Geometry check sheet. Reference: the model listing, model coordinates, mm. Face numbers are marked on the shaded views. Coordinates: 2 decimals unless noted, no trailing zeros. Loops run counter-clockwise (first coordinate to the right, second up) from the corner with the lowest first, then second, coordinate; pieces in that order, holes last.
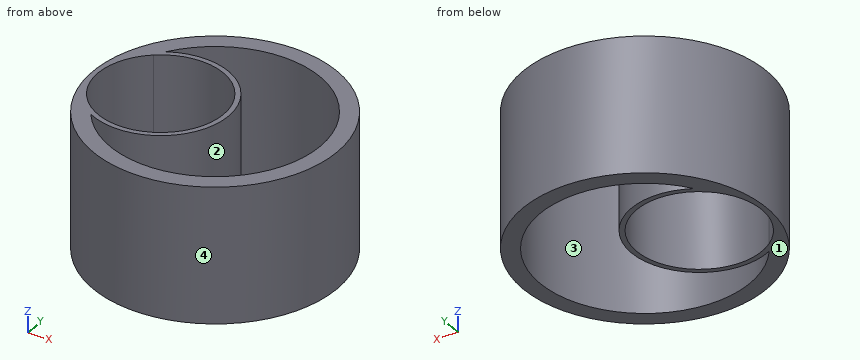
Autodesk Inventor part; units mm, degrees
ref_plane "YZ Plane" through (0, 0, 0) normal (1, 0, 0) x (0, 1, 0)
ref_plane "XZ Plane" through (0, 0, 0) normal (0, 1, 0) x (-1, 0, 0)
ref_plane "XY Plane" through (0, 0, 0) normal (0, 0, 1) x (1, 0, 0)
sketch "Sketch1" plane through (0, 0, 0) normal (0, 0, 1) x (1, 0, 0)
  line L0 (-6.35, 0) -> (-14.7828, 0) construction
  line L1 (0, 0) -> (30.9372, 0) construction
  circle A0 centre (30.9372, 0) radius 45.72
  line L2 (-14.7828, 0) -> (10.6172, 0) construction
  arc A1 (-1.4875, -22.3302) -> (-1.4875, 22.3302) centre (10.6172, 0) ccw
  arc A2 (-3.7794, -18.5675) -> (-3.7794, 18.5675) centre (10.6172, 0) ccw
  arc A3 (-1.4875, -22.3302) -> (-1.4875, 22.3302) centre (30.9372, 0) ccw
  arc A4 (-3.7794, 18.5675) -> (-3.7794, -18.5675) centre (10.6172, 0) ccw
  dimension "d1" = 8.4328
  dimension "d2" = 30.9372
  dimension "d6" = 25.4
  dimension "d7" = 46.99
extrude "Extrusion1" add sketch "Sketch1" along normal blind 50.8
properties part number "RO mark final"
(1) Sectioned sample at A-A on y = 0. Record the cut outline in (x, z).
Findings:
outline: (-14.78, 0) - (-12.88, 0) - (-12.88, 50.8) - (-14.78, 50.8) - close; (34.11, 0) - (36.02, 0) - (36.02, 50.8) - (34.11, 50.8) - close; (70.31, 0) - (76.66, 0) - (76.66, 50.8) - (70.31, 50.8) - close
(2) Gauge pin test, flat ends, axial feed: pin 1 Ø3 at (x, z) = (19, 11.5) entering from -Y; pin 2 Ø12 at (y, z) = (-8, 32.5) entering from -X; pin 3 Ø4 at (x, z) = (67.5, 17.5) entering from +Y. Record the tip position at first contact, or that the pin passes through.
Findings:
pin 1: stops at y = -44.51
pin 2: stops at x = -14.74
pin 3: stops at y = 29.93
(3) Scan lines: L1, parallel to X at y = -10.5, z = 3; L2, parallel to Y at x = 19.5, z = 9; L3, parallel to X at y = 21, z = 30. Record each from-to range of solid material in increasing order.
Findings:
L1: x = -13.56 to -10.4, 31.64 to 33.75, 68.88 to 75.44
L2: y = -44.27 to -37.67, -23.8 to -21.75, 21.75 to 23.8, 37.67 to 44.27
L3: x = -9.67 to 0.08, 21.15 to 24.91, 64.24 to 71.55
(4) Sectioned sample at D-D on x = -7. Record the cut outline in (y, z), and give its area (3 significant figures).
Findings:
outline: (-25.52, 0) - (-15.55, 0) - (-15.55, 50.8) - (-25.52, 50.8) - close; (15.55, 0) - (25.52, 0) - (25.52, 50.8) - (15.55, 50.8) - close
area: 1,010 mm2
(5) Sectioned sample at C-C on y = -37.5. Record the cut outline in (x, z), and give its area (3 significant figures).
Findings:
outline: (4.78, 0) - (18.95, 0) - (18.95, 50.8) - (4.78, 50.8) - close; (42.93, 0) - (57.09, 0) - (57.09, 50.8) - (42.93, 50.8) - close
area: 1,440 mm2
(6) Draft check along Y on the marked faces 1, 2, 3 and 4. Enter one of: +Y half, -Y half, draft (parallel to the pull), parting line (faces both ways), or undercut.
Findings:
face 1: draft
face 2: undercut
face 3: undercut
face 4: parting line
(7) Sectioned sample at B-B on x = 12. Record the cut outline in (y, z), and give its area (3 significant figures).
Findings:
outline: (-41.61, 0) - (-34.52, 0) - (-34.52, 50.8) - (-41.61, 50.8) - close; (-25.36, 0) - (-23.45, 0) - (-23.45, 50.8) - (-25.36, 50.8) - close; (23.45, 0) - (25.36, 0) - (25.36, 50.8) - (23.45, 50.8) - close; (34.52, 0) - (41.61, 0) - (41.61, 50.8) - (34.52, 50.8) - close
area: 915 mm2
